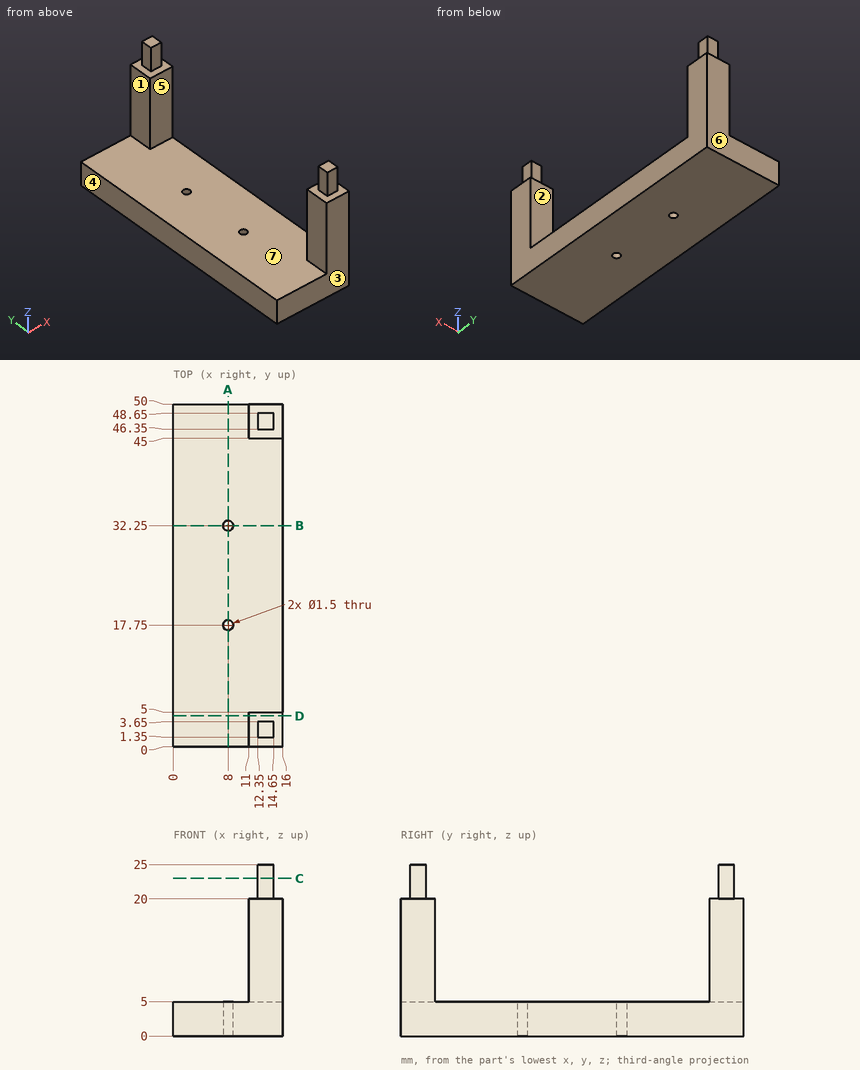
Source: three-view drawing plus pictorial views. Frame: mm from the lowest corner of the part. A direction names the side the tool comes from. Coordinates: 2 decimals unless noted, no trailing zeros. Write each loop counter-clockwise with the first axis right and the second up, starting at its lowest first coordinate (ties: lowest second). Pieces come first, ordered by that corner, then holes. Notation, with made-up numbers: (42.5, -3) -> (84.5, -3) arc R29 cw to (84.5, 21) -> close; hole circle Ø9 at (76, 46.25). An arc over 180 degrees is marked (long way). Answer as a JSON object with one key per item and string values.
1. Access query for the marked faces 1, 2 and 3. Directions: +Z, -Z, +X, -X, +Y, -Y. A direction counts if a zero-diameter tool reaches every point of the face in a straight line with its end or side. Return the directions, or none.
Result set:
{"face 1": "+Z, -X, +Y, -Y", "face 2": "+Z, +X, -X", "face 3": "+Z, -Z, +X, -X, -Y"}
2. First-contact query: P1, Ø1.2, axis at x = 13, z = 21.5, coming from the +Y side; P2, Ø6, axis at x = 6, z = 16.5, coming from the -Y side; P3, Ø2.5, axis at y = 2, z = 23.5, coming from the +X side; P4, Ø1.8, axis at x = 13.5, z = 22.5, coming from the -Y side. Flat tips, straight axial feed; report the tip coordinate or a pass-through.
Result set:
{"P1": "stops at y = 48.65", "P2": "passes through", "P3": "stops at x = 14.65", "P4": "stops at y = 1.35"}
3. Section A-A on x = 8. Return the cut outline in (y, z), then the cut area to 3 significant figures.
Result set:
{"outline": "(0, 0) -> (17, 0) -> (17, 5) -> (0, 5) -> close; (18.5, 0) -> (31.5, 0) -> (31.5, 5) -> (18.5, 5) -> close; (33, 0) -> (50, 0) -> (50, 5) -> (33, 5) -> close", "area": "235 mm2"}
4. Material intervals for line 1 (Y direction, x = 8, z = 3.05); line 2 (X direction, y = 17.75, z = 3.2); line 3 (Y direction, x = 13.75, z = 21), sorted ascending. Write a range as from..to.
Result set:
{"line 1": "y = 0..17, 18.5..31.5, 33..50", "line 2": "x = 0..7.25, 8.75..16", "line 3": "y = 1.35..3.65, 46.35..48.65"}
5. Mould query, pull axis Y, two halves, no side actions, for the marked faces 4, 5, 6 and 7. Classes: released by +Y, released by -Y, zero draft, split by the parting line, or undercut.
Result set:
{"face 4": "zero draft", "face 5": "undercut", "face 6": "released by +Y", "face 7": "undercut"}
6. Section C-C on z = 23. Return the cut outline in (x, y).
Result set:
{"outline": "(12.35, 1.35) -> (14.65, 1.35) -> (14.65, 3.65) -> (12.35, 3.65) -> close; (12.35, 46.35) -> (14.65, 46.35) -> (14.65, 48.65) -> (12.35, 48.65) -> close"}
7. Section B-B on y = 32.25. Return the cut outline in (x, z).
Result set:
{"outline": "(0, 0) -> (7.25, 0) -> (7.25, 5) -> (0, 5) -> close; (8.75, 0) -> (16, 0) -> (16, 5) -> (8.75, 5) -> close"}
8. Section D-D on y = 4.5. Return the cut outline in (x, z), then the cut area to 3 significant figures.
Result set:
{"outline": "(0, 0) -> (16, 0) -> (16, 20) -> (11, 20) -> (11, 5) -> (0, 5) -> close", "area": "155 mm2"}
